Check sheet for the modelled part. Datum: model origin and axes. Units: mm. Face numbers are marked on the shaded views. A direction names the side the tool comes from. Round coordinates to 2 decimals unless told otherwise and drop trailing zeros. Write each loop counter-clockwise with the first axis right and the second up, starting at its lowest first coordinate (ties: lowest second). Pieces come first, ordered by that corner, then holes. Notation, with made-up numbers: M 19,-19 L 24,-19 A13 cw 24,5 Z; hole C 41.5,23.5 d7. An arc over 180 degrees is marked long. One line per item, written item: value.
from build123d import *

# Parameters (mm, degrees)
BOSS_EXTRUDE1_DEPTH = 10
FILLET1_R           = 1
FILLET2_R           = 0.5


with BuildPart() as part:
    # Sketch1 → Boss-Extrude1 (new body)
    with BuildSketch(Plane(origin=(0, 0, 0), x_dir=(1, 0, 0), z_dir=(0, 1, 0))):
        Polygon((-8.118577075, -4.9), (-8.118577075, -6.9), (10.118577075, -5.776825706), (10.118577075, 9.9), (-8.118577075, 9.9), (-8.118577075, 7.9), (8.118577075, 7.9), (8.118577075, -3.3), align=None)
    extrude(amount=BOSS_EXTRUDE1_DEPTH)

    # Fillet1
    fillet1_edges = [part.edges().sort_by_distance(p)[0] for p in [
        (1, 0, -9.9),
        (10.118577075, 0, -2.061587147),
        (1, 0, 6.338412853),
        (-8.118577075, 5, -9.9),
        (10.118577075, 5, -9.9),
        (10.118577075, 5, 5.776825706),
        (-8.118577075, 5, 6.9),
        (1, 10, 6.338412853),
        (10.118577075, 10, -2.061587147),
        (1, 10, -9.9),
    ]]
    fillet(fillet1_edges, radius=FILLET1_R)

    # Fillet2
    fillet2_edges = [part.edges().sort_by_distance(p)[0] for p in [
        (8.118577075, 5, -7.9),
        (8.118577075, 5, 3.3),
    ]]
    fillet(fillet2_edges, radius=FILLET2_R)


solid = part.part
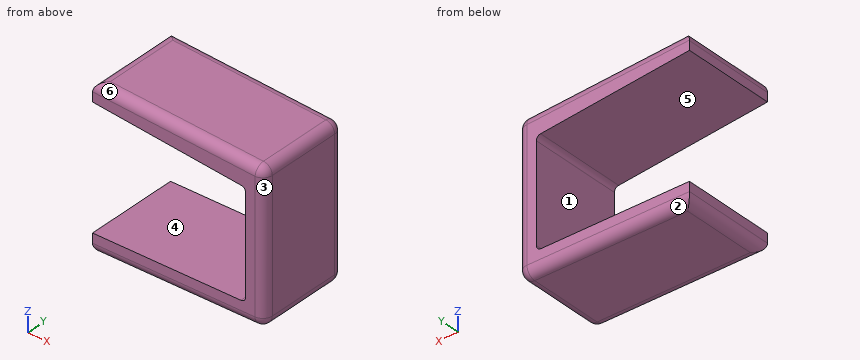
Q1. Depth check by flat-ended pin: P1, Ø5, axis at y = 7.5, z = -2.5, coming from the -X side; P2, Ø1.5, axis at x = 4.5, y = 3.5, coming from the +Z side; P3, Ø4, axis at x = -2, z = 2, coming from the -Y side; P4, Ø3, axis at x = -0.5, y = 6, coming from the +Z side. Enter the tip coordinate at first touch or a pass-through.
Completed:
P1: x = 8.12
P2: z = 6.17
P3: through
P4: z = 6.52
Q2. Access from +Z, -Z, +X, -X, +Y, -Y to the whole of each face (thin tool, end or side, straight path). Record for the marked faces 5 and 6.
Completed:
face 5: -X, +Y, -Y
face 6: +Z, +X, -Y
Q3. Sectioned sample at C-C on z = 4.5. Enter the section's corners in (x, y).
Completed:
outline: M -4.06,0 L 9.12,0 A1 ccw 10.12,1 L 10.12,9 A1 ccw 9.12,10 L -4.06,10 Z
Q4. Sectioned sample at B-B on z = 1. Enter the section's corners in (x, y).
Completed:
outline: M 8.12,0 L 9.12,0 A1 ccw 10.12,1 L 10.12,9 A1 ccw 9.12,10 L 8.12,10 Z
Q5. Scan lines: line 1 (X direction, y = 4, z = -6.25); line 2 (Z direction, x = -3.5, y = 7.5); line 3 (Z direction, x = 5.75, y = 8.5). Record each from-to range of solid material in increasing order. Write a range as [from, to].
Completed:
line 1: [8.12, 10.12]
line 2: [-9.9, -7.9], [4.44, 6.62]
line 3: [-9.9, -7.9], [3.53, 6.05]
Q6. Sectioned sample at A-A on y = 3.75. Enter the section's corners in (x, z), and give its area (3 significant figures).
Completed:
outline: M -8.12,-8.9 A1 ccw -7.12,-9.9 L 9.12,-9.9 A1 ccw 10.12,-8.9 L 10.12,4.84 A1 ccw 9.18,5.83 L -7.06,6.83 A1 ccw -8.12,5.84 L -8.12,4.9 L 7.67,3.34 A0.5 cw 8.12,2.85 L 8.12,-7.4 A0.5 cw 7.62,-7.9 L -8.12,-7.9 Z
area: 101 mm^2
Q7. Draft check along Z on the marked faces 1, 2, 3 and 4. Enter one of: pulls with the +Z half, pulls with the -Z half, needs draft (parallel to the pull), parting line crosses it, or undercut.
Completed:
face 1: undercut
face 2: pulls with the -Z half
face 3: needs draft
face 4: undercut
